from build123d import *

# Parameters (mm, degrees)
EXTRUDE_1_DEPTH     = 400
CUT_EXTRUDE_START   = -250
CUT_EXTRUDE_1_DEPTH = 250
SKETCH_3_R          = 15.665420251
SKETCH_3_R_2        = 18.510518013
CUT_EXTRUDE_2_DEPTH = 50
FILLET_2_R          = 90
FILLET_3_R          = 90
EXTRUDE_START       = 50
SKETCH_4_R          = 18.510518013
SKETCH_4_R_2        = 15.665420251
EXTRUDE_2_DEPTH     = 50
SKETCH_8_R          = 25
CUT_EXTRUDE_3_DEPTH = 100


with BuildPart() as part:
    # 草图1 → 凸台-拉伸1 (new body)
    with BuildSketch(Plane(origin=(0, 0, 0), x_dir=(1, 0, 0), z_dir=(0, 1, 0))):
        with BuildLine():
            ThreePointArc((1355.07847299, 407.415429308), (1351.426521797, 419.370189907), (1347.669105677, 431.292222979))
            ThreePointArc((1347.669105677, 431.292222979), (1331.935587475, 477.674147112), (1314.606303382, 523.483779222))
            Line((1314.606303382, 523.483779222), (1407.51134249, 560.479099308))
            Line((1407.51134249, 560.479099308), (1430.737602267, 569.72792933))
            Line((1430.737602267, 569.72792933), (1523.642641375, 606.723249416))
            ThreePointArc((1523.642641375, 606.723249416), (1566.317664839, 486.054495722), (1599.452391748, 362.425228886))
            Line((1599.452391748, 362.425228886), (1501.924806885, 340.326129564))
            Line((1501.924806885, 340.326129564), (1477.542910669, 334.801354733))
            Line((1477.542910669, 334.801354733), (1380.015325807, 312.702255411))
            ThreePointArc((1380.015325807, 312.702255411), (1368.366605987, 360.27466136), (1355.07847299, 407.415429308))
        make_face()
    extrude(amount=EXTRUDE_1_DEPTH)

    # 草图2 → 切除-拉伸1 (cut)
    with BuildSketch(Plane(origin=(0, 400, 0), x_dir=(1, 0, 0), z_dir=(0, 1, 0)).offset(CUT_EXTRUDE_START)):
        with BuildLine():
            Line((1347.669105677, 431.292222979), (1443.179761176, 460.930772385))
            ThreePointArc((1443.179761176, 460.930772385), (1426.214363088, 511.016233129), (1407.51134249, 560.479099308))
            Line((1407.51134249, 560.479099308), (1430.737602267, 569.72792933))
            ThreePointArc((1430.737602267, 569.72792933), (1470.810490154, 456.417026471), (1501.924806885, 340.326129564))
            Line((1501.924806885, 340.326129564), (1477.542910669, 334.801354733))
            ThreePointArc((1477.542910669, 334.801354733), (1464.958432674, 386.162906732), (1450.589128489, 437.053978714))
            Line((1450.589128489, 437.053978714), (1355.07847299, 407.415429308))
            ThreePointArc((1355.07847299, 407.415429308), (1351.426521797, 419.370189907), (1347.669105677, 431.292222979))
        make_face()
    extrude(amount=CUT_EXTRUDE_1_DEPTH, mode=Mode.SUBTRACT)

    # 草图3 → 切除-拉伸2 (cut)
    with BuildSketch(Plane.XZ):
        with Locations(Location((1537.673756185, -404.548414334, 0), (0, 0, 270))):
            Circle(SKETCH_3_R)
        with Locations(Location((1496.563725778, -537.026083805, 0), (0, 0, 270))):
            Circle(SKETCH_3_R_2)
    extrude(amount=-CUT_EXTRUDE_2_DEPTH, mode=Mode.SUBTRACT)

    # 圆角2
    fillet_2_edges = [part.edges().sort_by_distance(p)[0] for p in [
        (1523.642641375, 200, -606.723249416),
        (1599.452391748, 200, -362.425228886),
        (1566.317664839, 400, -486.054495722),
    ]]
    fillet(fillet_2_edges, radius=FILLET_2_R)

    # 圆角3
    # the kernel refuses this fillet: 90 mm, written as the material it takes off along each edge
    with BuildSketch(Plane(origin=(0, 400, 0), x_dir=(0.9886635459067241, 0, -0.15014790373209708), z_dir=(0.15014790373209708, 0, 0.9886635459067241))) as fillet_3_piece_1_section:
        with BuildLine():
            CenterArc((1415 + FILLET_3_R, -FILLET_3_R), FILLET_3_R, 90, 90)
            Line((1415 + FILLET_3_R, 0), (1415 + FILLET_3_R, FILLET_3_R * 0.02))
            Line((1415 + FILLET_3_R, FILLET_3_R * 0.02), (1415 - FILLET_3_R * 0.02, FILLET_3_R * 0.02))
            Line((1415 - FILLET_3_R * 0.02, FILLET_3_R * 0.02), (1415 - FILLET_3_R * 0.02, -FILLET_3_R))
            Line((1415 - FILLET_3_R * 0.02, -FILLET_3_R), (1415, -FILLET_3_R))
        make_face()
    fillet_3_piece_1 = revolve(axis=Axis((0, 400, 0), (0, 1, 0)), revolution_arc=13.077233198, mode=Mode.PRIVATE)
    fillet_3_piece_1 = split(fillet_3_piece_1, bisect_by=Plane(origin=(1365.899074688, 379.798837266, -436.949286418), z_dir=(-0.2963746925135586, 0, -0.9550717468533417)), keep=Keep.TOP, mode=Mode.PRIVATE)
    add(fillet_3_piece_1, mode=Mode.SUBTRACT)
    with BuildSketch(Plane(origin=(1696.97997661, 400, -384.524328208), x_dir=(0, -1, 0), z_dir=(-0.9752758486265656, 0, 0.22099099322310048))) as fillet_3_piece_2_section:
        with BuildLine():
            CenterArc((FILLET_3_R, -FILLET_3_R), FILLET_3_R, 90, 90)
            Line((0, -FILLET_3_R), (-FILLET_3_R * 0.02, -FILLET_3_R))
            Line((-FILLET_3_R * 0.02, -FILLET_3_R), (-FILLET_3_R * 0.02, FILLET_3_R * 0.02))
            Line((-FILLET_3_R * 0.02, FILLET_3_R * 0.02), (FILLET_3_R, FILLET_3_R * 0.02))
            Line((FILLET_3_R, FILLET_3_R * 0.02), (FILLET_3_R, 0))
        make_face()
    fillet_3_piece_2 = extrude(amount=550, mode=Mode.PRIVATE)
    fillet_3_piece_2 = fillet_3_piece_2 - Plane(origin=(0, 379.627251668, 0), x_dir=(0.9752758486265642, 0, -0.22099099322310606), z_dir=(0, -1, 0)) * Cylinder(1415, 1461, mode=Mode.PRIVATE)
    fillet_3_piece_2 = fillet_3_piece_2 & Plane(origin=(0, 379.627251668, 0), x_dir=(0.9752758486265641, 0, -0.22099099322310678), z_dir=(0, -1, 0)) * Cylinder(1515, 1461, mode=Mode.PRIVATE)
    add(fillet_3_piece_2, mode=Mode.SUBTRACT)
    with BuildSketch(Plane(origin=(1105.569965388, 400, -440.244309028), x_dir=(0, -1, 0), z_dir=(0.9290503910825915, 0, -0.36995320086368216))) as fillet_3_piece_3_section:
        with BuildLine():
            CenterArc((FILLET_3_R, -FILLET_3_R), FILLET_3_R, 90, 90)
            Line((0, -FILLET_3_R), (-FILLET_3_R * 0.02, -FILLET_3_R))
            Line((-FILLET_3_R * 0.02, -FILLET_3_R), (-FILLET_3_R * 0.02, FILLET_3_R * 0.02))
            Line((-FILLET_3_R * 0.02, FILLET_3_R * 0.02), (FILLET_3_R, FILLET_3_R * 0.02))
            Line((FILLET_3_R, FILLET_3_R * 0.02), (FILLET_3_R, 0))
        make_face()
    fillet_3_piece_3 = extrude(amount=550, mode=Mode.PRIVATE)
    fillet_3_piece_3 = fillet_3_piece_3 - Plane(origin=(0, 379.627145312, 0), x_dir=(0.9752758486265642, 0, -0.22099099322310606), z_dir=(0, -1, 0)) * Cylinder(1415, 1461, mode=Mode.PRIVATE)
    fillet_3_piece_3 = fillet_3_piece_3 & Plane(origin=(0, 379.627145312, 0), x_dir=(0.9525939017664254, 0, -0.30424473424764115), z_dir=(0, -1, 0)) * Cylinder(1515, 1461, mode=Mode.PRIVATE)
    add(fillet_3_piece_3, mode=Mode.SUBTRACT)
    with BuildSketch(Plane(origin=(0, 400, 0), x_dir=(0.9752758486265642, 0, -0.22099099322310606), z_dir=(0.22099099322310606, 0, 0.9752758486265642))) as fillet_3_piece_4_section:
        with BuildLine():
            CenterArc((1415 + FILLET_3_R, -FILLET_3_R), FILLET_3_R, 90, 90)
            Line((1415 + FILLET_3_R, 0), (1415 + FILLET_3_R, FILLET_3_R * 0.02))
            Line((1415 + FILLET_3_R, FILLET_3_R * 0.02), (1415 - FILLET_3_R * 0.02, FILLET_3_R * 0.02))
            Line((1415 - FILLET_3_R * 0.02, FILLET_3_R * 0.02), (1415 - FILLET_3_R * 0.02, -FILLET_3_R))
            Line((1415 - FILLET_3_R * 0.02, -FILLET_3_R), (1415, -FILLET_3_R))
        make_face()
    fillet_3_piece_4 = revolve(axis=Axis((0, 400, 0), (0, 1, 0)), revolution_arc=13.077233198, mode=Mode.PRIVATE)
    fillet_3_piece_4 = split(fillet_3_piece_4, bisect_by=Plane(origin=(1373.308440607, 379.798836933, -413.072492314), z_dir=(0.29637469251355963, 0, 0.9550717468533415)), keep=Keep.TOP, mode=Mode.PRIVATE)
    add(fillet_3_piece_4, mode=Mode.SUBTRACT)
    with BuildSketch(Plane(origin=(0, 400, 0), x_dir=(0.9886635459067241, 0, -0.15014790373209708), z_dir=(0.15014790373209708, 0, 0.9886635459067241))) as fillet_3_piece_5a_section:
        with BuildLine():
            CenterArc((1415 + FILLET_3_R, -FILLET_3_R), FILLET_3_R, 90, 90)
            Line((1415 + FILLET_3_R, 0), (1415 + FILLET_3_R, FILLET_3_R * 0.02))
            Line((1415 + FILLET_3_R, FILLET_3_R * 0.02), (1415 - FILLET_3_R * 0.02, FILLET_3_R * 0.02))
            Line((1415 - FILLET_3_R * 0.02, FILLET_3_R * 0.02), (1415 - FILLET_3_R * 0.02, -FILLET_3_R))
            Line((1415 - FILLET_3_R * 0.02, -FILLET_3_R), (1415, -FILLET_3_R))
        make_face()
    fillet_3_piece_5a = revolve(axis=Axis((0, 400, 0), (0, 1, 0)), revolution_arc=22.187876624, mode=Mode.PRIVATE)
    fillet_3_piece_5a = split(fillet_3_piece_5a, bisect_by=Plane(origin=(1328.166352614, 379.779381403, -528.883468696), z_dir=(-0.3699532008636821, 0, -0.9290503910825915)), keep=Keep.TOP, mode=Mode.PRIVATE)
    with BuildSketch(Plane(origin=(1105.569965388, 400, -440.244309028), x_dir=(0, -1, 0), z_dir=(0.9290503910825915, 0, -0.36995320086368216))) as fillet_3_piece_5b_section:
        with BuildLine():
            CenterArc((FILLET_3_R, -FILLET_3_R), FILLET_3_R, 90, 90)
            Line((0, -FILLET_3_R), (-FILLET_3_R * 0.02, -FILLET_3_R))
            Line((-FILLET_3_R * 0.02, -FILLET_3_R), (-FILLET_3_R * 0.02, FILLET_3_R * 0.02))
            Line((-FILLET_3_R * 0.02, FILLET_3_R * 0.02), (FILLET_3_R, FILLET_3_R * 0.02))
            Line((FILLET_3_R, FILLET_3_R * 0.02), (FILLET_3_R, 0))
        make_face()
    fillet_3_piece_5b = extrude(amount=550, mode=Mode.PRIVATE)
    fillet_3_piece_5b = fillet_3_piece_5b & Plane(origin=(0, 379.605879508, 0), x_dir=(0.9752758486265642, 0, -0.22099099322310606), z_dir=(0, -1, 0)) * Cylinder(1415, 1461, mode=Mode.PRIVATE)
    fillet_3_piece_5 = fillet_3_piece_5a & fillet_3_piece_5b
    add(fillet_3_piece_5, mode=Mode.SUBTRACT)
    with BuildSketch(Plane(origin=(1696.97997661, 400, -384.524328208), x_dir=(0, -1, 0), z_dir=(-0.9752758486265656, 0, 0.22099099322310048))) as fillet_3_piece_6a_section:
        with BuildLine():
            CenterArc((FILLET_3_R, -FILLET_3_R), FILLET_3_R, 90, 90)
            Line((0, -FILLET_3_R), (-FILLET_3_R * 0.02, -FILLET_3_R))
            Line((-FILLET_3_R * 0.02, -FILLET_3_R), (-FILLET_3_R * 0.02, FILLET_3_R * 0.02))
            Line((-FILLET_3_R * 0.02, FILLET_3_R * 0.02), (FILLET_3_R, FILLET_3_R * 0.02))
            Line((FILLET_3_R, FILLET_3_R * 0.02), (FILLET_3_R, 0))
        make_face()
    fillet_3_piece_6a = extrude(amount=550, mode=Mode.PRIVATE)
    fillet_3_piece_6a = fillet_3_piece_6a & Plane(origin=(0, 379.60590325, 0), x_dir=(0.9752758486265642, 0, -0.22099099322310606), z_dir=(0, -1, 0)) * Cylinder(1415, 1461, mode=Mode.PRIVATE)
    with BuildSketch(Plane(origin=(0, 400, 0), x_dir=(0.9979642112015443, 0, -0.06377643107668678), z_dir=(0.06377643107668678, 0, 0.9979642112015443))) as fillet_3_piece_6b_section:
        with BuildLine():
            CenterArc((1415 + FILLET_3_R, -FILLET_3_R), FILLET_3_R, 90, 90)
            Line((1415 + FILLET_3_R, 0), (1415 + FILLET_3_R, FILLET_3_R * 0.02))
            Line((1415 + FILLET_3_R, FILLET_3_R * 0.02), (1415 - FILLET_3_R * 0.02, FILLET_3_R * 0.02))
            Line((1415 - FILLET_3_R * 0.02, FILLET_3_R * 0.02), (1415 - FILLET_3_R * 0.02, -FILLET_3_R))
            Line((1415 - FILLET_3_R * 0.02, -FILLET_3_R), (1415, -FILLET_3_R))
        make_face()
    fillet_3_piece_6b = revolve(axis=Axis((0, 400, 0), (0, 1, 0)), revolution_arc=22.187876624, mode=Mode.PRIVATE)
    fillet_3_piece_6b = split(fillet_3_piece_6b, bisect_by=Plane(origin=(1394.250064092, 379.779381346, -315.927752029), z_dir=(0.22099099322310004, 0, 0.9752758486265657)), keep=Keep.TOP, mode=Mode.PRIVATE)
    fillet_3_piece_6 = fillet_3_piece_6a & fillet_3_piece_6b
    add(fillet_3_piece_6, mode=Mode.SUBTRACT)

    # 草图4 → 凸台-拉伸2 (add)
    with BuildSketch(Plane.XZ.offset(-50).offset(EXTRUDE_START)):
        with Locations((1496.563725778, -537.026083805)):
            Circle(SKETCH_4_R)
        with Locations((1537.673756185, -404.548414334)):
            Circle(SKETCH_4_R_2)
    extrude(amount=-EXTRUDE_2_DEPTH)

    # 草图8 → 切除-拉伸3 (cut)
    with BuildSketch(Plane.XZ):
        with Locations(Location((1431.534758427, -375.643761315, 0), (0, 0, 270))):
            Circle(SKETCH_8_R)
        with Locations(Location((1392.707343884, -500.765668043, 0), (0, 0, 270))):
            Circle(SKETCH_8_R)
    extrude(amount=-CUT_EXTRUDE_3_DEPTH, mode=Mode.SUBTRACT)


solid = part.part
The listing builds one solid part. Answer for the finished solid, in the listing's coordinates (mm). A direction names the side the tool comes from. Round coordinates to 2 decimals unless told otherwise and drop trailing zeros. Write each loop counter-clockwise with the first axis right and the second up, starting at its lowest first coordinate (ties: lowest second). Pieces come first, ordered by that corner, then holes. Notation, with made-up numbers: M 83,-31.5 L 131,-31.5 A33 cw 131,5.5 Z; hole C -34.75,-19 d10. An arc over 180 degrees is marked long. Write each question's results on one line, items separated by ' | '. Start each with the question number.
Item 1: Find section B-B on y = 70. Write down the section's boundary in (x, z), and give its area (3 significant figures).
Item 2: The mould has two halves that part along Z. Classify faces 4 (the cylindrical face through (1566.182, 152.83, -486.492)), 5 (the flat face through (1436, 400, -467)), 6 (the cylindrical face through (1452.615, 49.3, -389.084)): +Z half, -Z half, draft (parallel to the pull), parting line (faces both ways), or undercut.
Item 3: Find section C-C on y = 336.5. Write down the section's boundary in (x, z).
Item 4: Given pin 1 Ø10 at (y, z) = (80.5, -520) entering from +X; pin 2 Ø1 at (x, z) = (1417, -342) entering from +Y; pin 3 Ø3 at (x, z) = (1507, -401.5) entering from -Y; pin 4 Ø5 at (x, z) = (1424, -425) entering from +Y, each flat-ended and moving along its own axis, determine where each tip first touches the part or whether it passes through.
Item 5: Find section A-A on y = 292.5. Write down the section's boundary in (x, z), and give its area (3 significant figures).
Item 6: Straight lines are drawn through the part: probe 1 along X at (y, z) = (310, -391); probe 2 along X at (y, z) = (367, -371); probe 3 along Y at (x, z) = (1384, -530.5). For each, find the intervals that lie inside material, in ascending order.
Item 7: Which of the six approach directions +Z, -Z, +X, -X, +Y, -Y give full straight-line access (tool end or side, diameter ignored) to faces 1 (the flat face through (1448, 400, -429)), 2 (the flat face through (1403.5, 273.25, -422.44)), 3 (the flat face through (1432, 100, -375))?
Answer block:
1) outline: M 1314.61,-523.48 L 1437.6,-572.46 A90 ccw 1556.3,-517.23 A1640 ccw 1575.71,-454.69 A90 ccw 1509.13,-341.96 L 1380.02,-312.7 A1415 cw 1355.08,-407.42 A1415 cw Z; hole C 1392.71,-500.77 d50; hole C 1431.53,-375.64 d50 | area: 45,900 mm²
2) face 4: -Z half | face 5: draft | face 6: undercut
3) outline: M 1319.78,-521.25 L 1408.98,-556.77 A1515 ccw 1443.18,-460.93 L 1351.48,-432.47 A1418.99 cw Z; M 1358.89,-408.6 L 1450.59,-437.05 A1515 ccw 1476.66,-338.69 L 1383.02,-317.47 A1418.99 cw Z; M 1430.74,-569.73 L 1437.6,-572.46 A90 ccw 1543.71,-541.74 A1636.01 ccw 1579.21,-427.36 A90 ccw 1509.13,-341.96 L 1501.92,-340.33 A1540 cw Z
4) pin 1: stops at x = 1557.04 | pin 2: stops at y = 367.66 | pin 3: stops at y = 0 | pin 4: stops at y = 398.49
5) outline: M 1314.61,-523.48 L 1407.51,-560.48 A1515 ccw 1443.18,-460.93 L 1347.67,-431.29 A1415 cw Z; M 1355.08,-407.42 L 1450.59,-437.05 A1515 ccw 1477.54,-334.8 L 1380.02,-312.7 A1415 cw Z; M 1430.74,-569.73 L 1437.6,-572.46 A90 ccw 1556.3,-517.23 A1640 ccw 1575.71,-454.69 A90 ccw 1509.13,-341.96 L 1501.92,-340.33 A1540 cw Z | area: 41,400 mm²
6) probe 1: x = 1359.91 to 1463.67, 1489.54 to 1570.48 | probe 2: x = 1386.58 to 1468.87, 1494.64 to 1557.43 | probe 3: y = 0 to 365.51
7) face 1: +Z, -Z, +X, -X, +Y | face 2: +Y | face 3: -Y
